from build123d import *

# Parameters (mm, degrees)
SKETCH1_R           = 7.14375
BOSS_EXTRUDE1_DEPTH = 3.175
BOSS_EXTRUDE3_START = -6.35
SKETCH2_R           = 7.14375
BOSS_EXTRUDE3_DEPTH = 6.35


with BuildPart() as part:
    # Sketch1 → Boss-Extrude1 (new, symmetric)
    with BuildSketch(Plane.XY):
        Polygon((-20.6375, 0), (20.6375, 0), (68.2625, -95.25), (68.2625, -136.525), (-68.2625, -136.525), (-68.2625, -95.25), align=None)
        with Locations((0, -115.8875)):
            Circle(SKETCH1_R, mode=Mode.SUBTRACT)
        with Locations((0, -68.2625)):
            Circle(SKETCH1_R, mode=Mode.SUBTRACT)
        with Locations((0, -20.6375)):
            Circle(SKETCH1_R, mode=Mode.SUBTRACT)
        with Locations((47.625, -115.8875)):
            Circle(SKETCH1_R, mode=Mode.SUBTRACT)
        with Locations((-47.625, -115.8875)):
            Circle(SKETCH1_R, mode=Mode.SUBTRACT)
    extrude(amount=BOSS_EXTRUDE1_DEPTH, both=True)

    # Sketch2 → Boss-Extrude3 (add)
    with BuildSketch(Plane.XY.offset(3.175).offset(BOSS_EXTRUDE3_START)):
        with Locations((0, -68.2625)):
            Circle(SKETCH2_R)
        with Locations((0, -20.6375)):
            Circle(SKETCH2_R)
        with Locations((-47.625, -115.8875)):
            Circle(SKETCH2_R)
        with Locations((0, -115.8875)):
            Circle(SKETCH2_R)
        with Locations((47.625, -115.8875)):
            Circle(SKETCH2_R)
    extrude(amount=BOSS_EXTRUDE3_DEPTH)


solid = part.part
Build history of the part. All positions in model axes, mm. Coordinates: 2 decimals unless noted, no trailing zeros. Order: outer loops, then holes, each group sorted by start corner. A loop starts at its lowest first (then second) coordinate and runs counter-clockwise, first axis right, second up. Notation, with made-up numbers: (62, 85) - (91, 85) arc R37 ccw to (91, 121) - close; hole circle Ø2 at (60.5, 12). An arc over 180 degrees is marked (long way). Write item = value, one per line. Start each with the question number.
1) Saw through at C-C on x = 34. Write the cut outline in (y, z) (3 decimals), then the cut area to 3 significant figures.
2) Flat gauge pins, fed straight in: pin 1 Ø3 at (y, z) = (-70.5, 2) entering from +X; pin 2 Ø1 at (y, z) = (-36, 0.5) entering from -X; pin 3 Ø1 at (y, z) = (-45, -1) entering from -X. Where does each tip first touch, or does it go through?
3) Saw through at B-B on y = -92.5. Write the cut outline in (x, z) (1 decimal).
4) Two-plate mould, pull along X, no slides. Class faces 1 (the face through (-44.783, -48.292, 0.044)), 2 (the face through (1, -82, 3.175)), 3 (the face through (68.262, -116, 0)): pulls with the +X half, pulls with the -X half, needs draft (parallel to the pull), parting line crosses it, or undercut.
5) Wall check: line 1 along Y through (x, z) = (28.5, 0.75) (3 decimals); line 2 along Y through (x, z) = (38, 0.25) (3 decimals); line 3 along X through (y, z) = (-58, 2). Give the ranges that are in metal, low to high. Write a range as from..to.
From the geometry:
q1.outline = (-136.525, -3.175) - (-26.725, -3.175) - (-26.725, 3.175) - (-136.525, 3.175) - close
q1.area = 697 mm^2
q2.pin_1 = 56.64
q2.pin_2 = -38.89
q2.pin_3 = -43.39
q3.outline = (-66.9, -3.2) - (66.9, -3.2) - (66.9, 3.2) - (-66.9, 3.2) - close
q4.face_1 = pulls with the -X half
q4.face_2 = needs draft
q4.face_3 = pulls with the +X half
q5.line_1 = -136.525..-15.725
q5.line_2 = -136.525..-34.725
q5.line_3 = -49.64..49.64
